For this review, take the finished solid that the model builds, in its own axes (mm). A direction names the side the tool comes from. Round coordinates to 2 decimals unless told otherwise and drop trailing zeros. Order: outer loops, then holes, each group sorted by start corner. A loop starts at its lowest first (then second) coordinate and runs counter-clockwise, first axis right, second up. Notation, with made-up numbers: (-9.5, 58) - (26.5, 58) arc R14 ccw to (26.5, 81) - close; hole circle Ø11 at (-26, -32.75). An arc over 180 degrees is marked (long way). One line per item, written item: value.
```python
from build123d import *

# Parameters (mm, degrees)
BOSS_EXTRUDE1_DEPTH = 18
SKETCH2_R           = 2
CUT_EXTRUDE1_DEPTH  = 48.391982444
SKETCH3_R           = 4
CUT_EXTRUDE2_DEPTH  = 44.703546936


with BuildPart() as part:
    # Sketch1 → Boss-Extrude1 (new body)
    with BuildSketch(Plane.XY):
        with BuildLine():
            Line((-31, 0), (-19, 0))
            ThreePointArc((-19, 0), (0, 19), (19, 0))
            Line((19, 0), (31, 0))
            ThreePointArc((31, 0), (0, 31), (-31, 0))
        make_face()
    extrude(amount=BOSS_EXTRUDE1_DEPTH)

    # Sketch2 → Cut-Extrude1 (cut, through all)
    with BuildSketch(Plane.XZ):
        with Locations(Location((-24.165982166, 9, 0), (0, 0, 270))):
            Circle(SKETCH2_R)
        with Locations(Location((25, 9, 0), (0, 0, 270))):
            Circle(SKETCH2_R)
    extrude(amount=-CUT_EXTRUDE1_DEPTH, mode=Mode.SUBTRACT)

    # Sketch3 → Cut-Extrude2 (cut, through all)
    with BuildSketch(Plane(origin=(0, 6, 0), x_dir=(1, 0, 0), z_dir=(0, 1, 0))):
        with Locations(Location((-24.165982166, -9, 0), (0, 0, 90))):
            Circle(SKETCH3_R)
        with Locations(Location((25, -9, 0), (0, 0, 90))):
            Circle(SKETCH3_R)
    extrude(amount=CUT_EXTRUDE2_DEPTH, mode=Mode.SUBTRACT)


solid = part.part
```
Item 1: Machinability: for faces 4 (the cylindrical face through (21.034, 12.417, 9.521)), 5 (the flat face through (-0.4, 19.2, 0)), which of the approach directions +Z, -Z, +X, -X, +Y, -Y give a long, thin tool a straight path to every point of the face, cutting with its end or side? Answer none if there is none.
Returned:
face 4: +Y
face 5: -Z, +X, -X, +Y, -Y
Item 2: For P1, Ø6.5, axis at x = 25, z = 9, coming from the +Y side; P2, Ø5, axis at y = 20.5, z = 13, coming from the +X side; P3, Ø3, axis at x = -19, z = 5.5, coming from the +Y side; P4, Ø3.5, axis at x = -24.17, z = 9, coming from the +Y side, all flat-tipped, find the tip position at first contact; note any pin that passes through.
Returned:
P1: y = 6
P2: x = 25.24
P3: y = 25.59
P4: through
Item 3: Take a section at B-B (y = 15). Write out the cut boundary in (x, z).
Returned:
outline: (-27.13, 0) - (-11.66, 0) - (-11.66, 18) - (-27.13, 18) - (-27.13, 11.69) arc R4 cw (long way) to (-27.13, 6.31) - close; (11.66, 0) - (27.13, 0) - (27.13, 5.61) arc R4 cw (long way) to (27.13, 12.39) - (27.13, 18) - (11.66, 18) - close
Item 4: Take a section at C-C (x = 25). Write out the cut boundary in (y, z), plus the area to 3 significant figures.
Returned:
outline: (0, 0) - (18.33, 0) - (18.33, 5) - (6, 5) - (6, 7) - (0, 7) - close; (0, 11) - (6, 11) - (6, 13) - (18.33, 13) - (18.33, 18) - (0, 18) - close
area: 207 mm^2
Item 5: Wall thickness on line 1 (X direction, y = 5, z = 9.75); line 2 (X direction, y = 3.45, z = 9); line 3 (X direction, y = 5.5, z = 12.25): over which ranges is each line inside the solid? List them lowest first.
Returned:
line 1: -30.59 to -26.02, -22.31 to -18.33, 18.33 to 23.15, 26.85 to 30.59
line 2: -30.81 to -26.17, -22.17 to -18.68, 18.68 to 23, 27 to 30.81
line 3: -30.51 to -18.19, 18.19 to 30.51
Item 6: Take a section at A-A (y = 5). Write out the cut boundary in (x, z), plus the area to 3 significant figures.
Returned:
outline: (-30.59, 0) - (-18.33, 0) - (-18.33, 18) - (-30.59, 18) - close; (18.33, 0) - (30.59, 0) - (30.59, 18) - (18.33, 18) - close; hole circle Ø4 at (-24.17, 9); hole circle Ø4 at (25, 9)
area: 416 mm^2
Item 7: The part is to be moulded in two halves that separate along Z. For faces 1 (the flat face through (-0.4, 19.2, 18)), 2 (the cylindrical face through (-22.183, 2.958, 9.26)), 3 (the flat face through (26, 0, 7)), say which applies: +Z half, -Z half, draft (parallel to the pull), parting line (faces both ways), or undercut.
Returned:
face 1: +Z half
face 2: undercut
face 3: draft
Item 8: Take a section at D-D (z = 9). Write out the cut boundary in (x, y), plus the area to 3 significant figures.
Returned:
outline: (-31, 0) - (-26.17, 0) - (-26.17, 6) - (-28.17, 6) - (-28.17, 12.95) arc R31 ccw to start; (-22.17, 0) - (-19, 0) arc R19 cw to (19, 0) - (23, 0) - (23, 6) - (21, 6) - (21, 22.8) arc R31 ccw to (-20.17, 23.54) - (-20.17, 6) - (-22.17, 6) - close; (27, 0) - (31, 0) arc R31 ccw to (29, 10.95) - (29, 6) - (27, 6) - close
area: 695 mm^2
